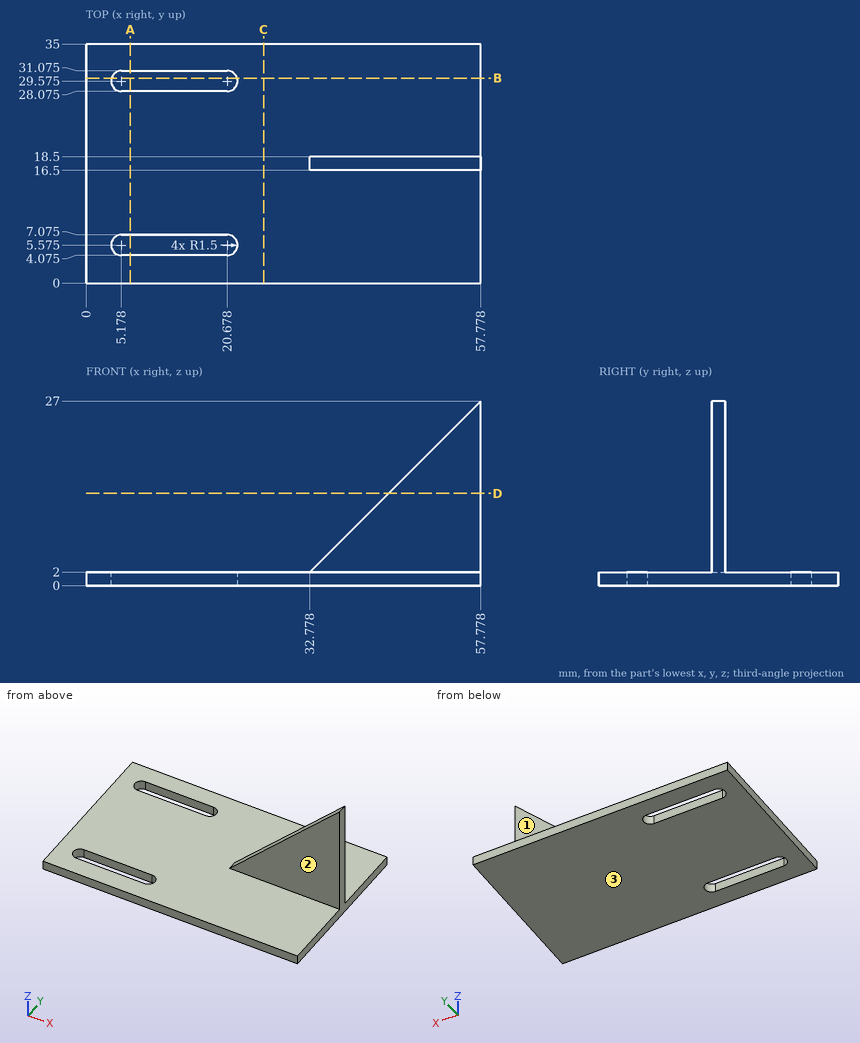
Source: three-view drawing plus pictorial views. Frame: mm from the lowest corner of the part. A direction names the side the tool comes from. Give positions to 0.01 mm unless a question says otherwise; leave off trailing zeros. Loops run counter-clockwise (first coordinate to the right, second up) from the corner with the lowest first, then second, coordinate; pieces in that order, holes last. Notation, with made-up numbers: M 61,28 L 117,28 A34 ccw 117,66 Z; hole C 24,8.25 d10. An arc over 180 degrees is marked long. Put each result on its own line as item: value.
Q1. Pin query (flat end, axial travel): P1, Ø10, axis at y = 9, z = 11.5, coming from the -X side; P2, Ø8, axis at y = 13, z = 4, coming from the +X side; P3, Ø10, axis at y = 20.5, z = 18, coming from the -X side (1 decimal); P4, Ø2, axis at x = 37.5, z = 5.5, coming from the +Y side. Return the tip coordinate at first contact, or that it passes through.
Response values:
P1: passes through
P2: stops at x = 57.78
P3: stops at x = 44.2
P4: stops at y = 18.5
Q2. Section D-D (z = 13.5). Return the cut outline in (x, y), and give its area (3 significant figures).
Response values:
outline: M 44.28,16.5 L 57.78,16.5 L 57.78,18.5 L 44.28,18.5 Z
area: 27.0 mm²
Q3. Section A-A (x = 6.5). Return the cut outline in (y, z) (3 decimals), and give its area (3 significant figures).
Response values:
outline: M 0,0 L 4.075,0 L 4.075,2 L 0,2 Z; M 7.075,0 L 28.075,0 L 28.075,2 L 7.075,2 Z; M 31.075,0 L 35,0 L 35,2 L 31.075,2 Z
area: 58.0 mm²
Q4. Reachability of the marked faces 1, 2 and 3 from +Z, -Z, +X, -X, +Y, -Y: full face, straight path, thin tool, end or side. Return the list, or none.
Response values:
face 1: +Z, +X, -X, +Y
face 2: +Z, +X, -X, -Y
face 3: -Z, +X, -X, +Y, -Y
Q5. Section B-B (y = 30). Return the cut outline in (x, z).
Response values:
outline: M 0,0 L 3.74,0 L 3.74,2 L 0,2 Z; M 22.12,0 L 57.78,0 L 57.78,2 L 22.12,2 Z
Q6. Line query: probe 1 along Z at (x, y) = (43, 28); probe 2 along Y at (x, z) = (54.5, 6.75); probe 3 along X at (y, z) = (17.5, 25.25). Output: solid intervals per line, ascending. Write a range as [from, to].
Response values:
probe 1: z = [0, 2]
probe 2: y = [16.5, 18.5]
probe 3: x = [56.03, 57.78]
Q7. Section C-C (x = 26). Return the cut outline in (y, z).
Response values:
outline: M 0,0 L 35,0 L 35,2 L 0,2 Z
